The listing builds one solid part. Answer for the finished solid, in the listing's coordinates (mm). A direction names the side the tool comes from. Give positions to 0.01 mm unless a question says otherwise; leave off trailing zeros. Write each loop counter-clockwise with the first axis right and the second up, starting at its lowest first coordinate (ties: lowest second). Pieces come first, ordered by that corner, then holes. Notation, with made-up numbers: (-12, 89) - (36, 89) arc R13 cw to (36, 109) - close; hole circle Ø1 at (-3.75, -20.5). An arc over 180 degrees is marked (long way). Return JSON: item names as keys, results as strings.
from build123d import *

# Parameters (mm, degrees)
F1_DEPTH = 19.05
F2_R     = 5
F3_R     = 1.5
F4_DEPTH = 2.6


with BuildPart() as f1:
    # F0 (on Front) → F1 (new body)
    with BuildSketch(Plane.XZ):
        with BuildLine():
            Line((3.3472654321, 31.1172038595), (2.0037624331, 32.4607068585))
            Line((2.0037624331, 32.4607068585), (-15.6739070966, 14.7830373289))
            ThreePointArc((-15.6739070966, 14.7830373289), (-16.6277072024, 9.9879603892), (-12.5626372594, 7.2717674916))
            Line((-12.5626372594, 7.2717674916), (37.4373627406, 7.2717674916))
            Line((37.4373627406, 7.2717674916), (37.4373627406, 9.1717676539))
            Line((37.4373627406, 9.1717676539), (-12.5626372594, 9.1717676539))
            ThreePointArc((-12.5626372594, 9.1717676539), (-14.8723359407, 10.7150589728), (-14.3304040976, 13.4395343299))
            Line((-14.3304040976, 13.4395343299), (3.3472654321, 31.1172038595))
        make_face()
    extrude(amount=F1_DEPTH)

    # F2
    f2_edges = [f1.edges().sort_by_distance(p)[0] for p in [
        (37.437363, -19.05, 8.221768),
        (37.437363, 0, 8.221768),
        (2.675514, -19.05, 31.788955),
        (2.675514, 0, 31.788955),
    ]]
    fillet(f2_edges, radius=F2_R)

    # F3 (on face) → F4 (cut)
    with BuildSketch(Plane(origin=(-15.2284722127, 0, 15.2284722127), x_dir=(0, -1, 0), z_dir=(-0.7071067812, 0, 0.7071067812))):
        with Locations((4.5, 16.8700599461)):
            Circle(F3_R)
        with Locations((14.55, 16.8700599461)):
            Circle(F3_R)
    extrude(amount=-F4_DEPTH, mode=Mode.SUBTRACT)


solid = f1.part
Item 1: A cutting plane is placed at B-B on y = -10.75. Determine the outline of the cut face in (x, z), then the cut area to 3 significant figures.
Answer below:
{"outline": "(-15.67, 14.78) arc R4.4 ccw to (-12.56, 7.27) - (37.44, 7.27) - (37.44, 9.17) - (-12.56, 9.17) arc R2.5 cw to (-14.33, 13.44) - (3.35, 31.12) - (2, 32.46) - close", "area": "158 mm²"}
Item 2: Consider L1, parallel to Z at x = 31, y = -2.75; L2, parallel to Z at x = -3.5, y = -8.25; L3, parallel to Z at x = -14, y = -12.75. Determine where each line is inside the solid, lowest interval first.
Answer below:
{"L1": "z = 7.27 to 9.17", "L2": "z = 7.27 to 9.17, 24.27 to 26.96", "L3": "z = 7.51 to 9.63, 13.77 to 16.46"}
Item 3: A cutting plane is placed at D-D on z = 10. Determine the outline of the cut face in (x, y).
Answer below:
{"outline": "(-16.63, -19.05) - (-14.42, -19.05) - (-14.42, 0) - (-16.63, 0) - close"}
Item 4: The mould has two halves that part along X. Classify faces 1 (the face through (12, -9, 7.272)), 2 (the face through (-2.32, -5.93, 26.81)), 3 (the face through (-5.62, -9.39, 22.15)): +X half, -X half, draft (parallel to the pull), parting line (faces both ways), or undercut.
Answer below:
{"face 1": "draft", "face 2": "undercut", "face 3": "+X half"}
Item 5: A cutting plane is placed at C-C on x = 16.5. Determine the outline of the cut face in (y, z), then the cut area to 3 significant figures.
Answer below:
{"outline": "(-19.05, 7.27) - (0, 7.27) - (0, 9.17) - (-19.05, 9.17) - close", "area": "36.2 mm²"}
Item 6: A cutting plane is placed at A-A on x = -5. Determine the outline of the cut face in (y, z), then the cut area to 3 significant figures.
Answer below:
{"outline": "(-19.05, 7.27) - (0, 7.27) - (0, 9.17) - (-19.05, 9.17) - close; (-19.05, 22.77) - (0, 22.77) - (0, 25.46) - (-19.05, 25.46) - close", "area": "87.4 mm²"}
Item 7: Flat-ended cylindrical pins translate along their axes: P1, Ø1.5, axis at y = -10.5, z = 22.5, coming from the -X side; P2, Ø4, axis at x = -6.5, y = -2, coming from the +Z side; P3, Ø10, axis at x = 25.5, y = -2.5, coming from the +Z side; P4, Ø5, axis at x = -1, z = 26.5, coming from the +Y side. Find the tip coordinate at first contact, or state that the pin passes through.
Answer below:
{"P1": "stops at x = -8.71", "P2": "stops at z = 25.96", "P3": "stops at z = 9.17", "P4": "stops at y = 0"}
Item 8: For faces 4 (the face through (37.437, -9, 8)), 5 (the face through (13, -9, 9.172)), determine the directions among +Z, -Z, +X, -X, +Y, -Y from which every point of the face is accessible in a straight line to the end or side of a thin tool.
Answer below:
{"face 4": "+Z, -Z, +X, +Y, -Y", "face 5": "+X, +Y, -Y"}
